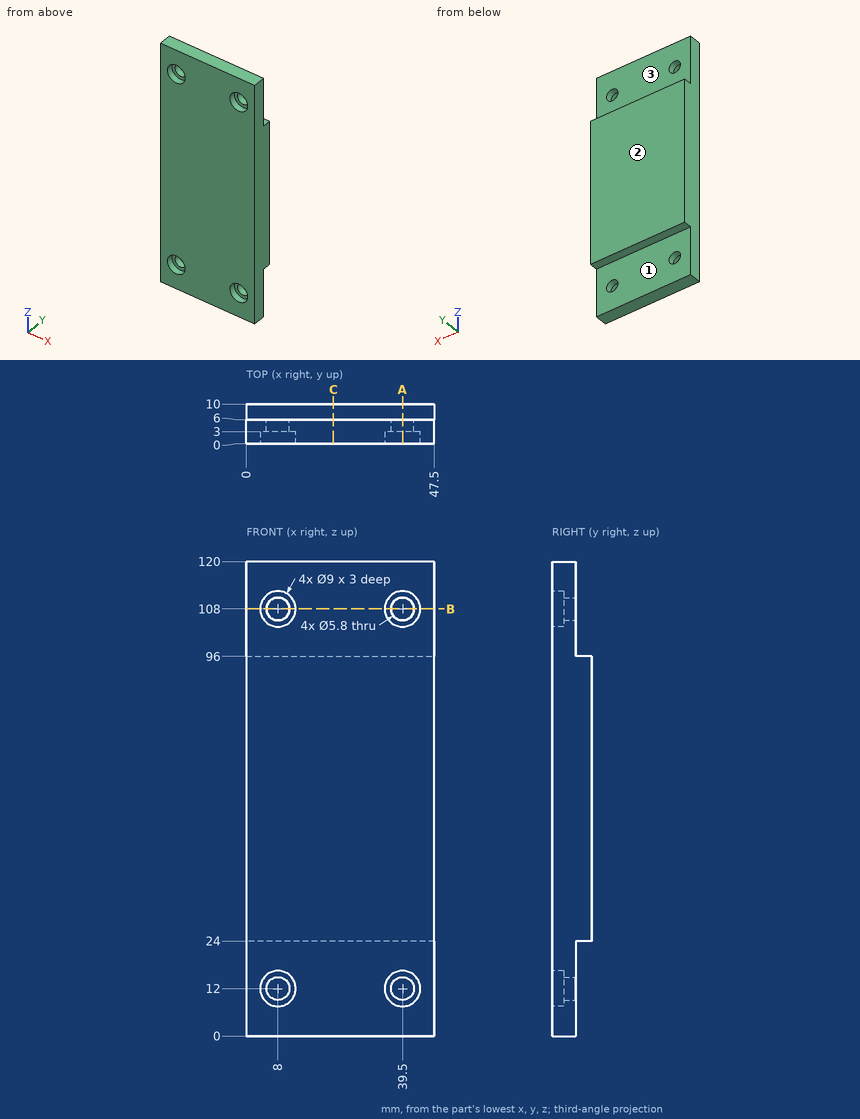
Job drawing, mm, ordinate dimensions from the low corner. One solid piece. A direction names the side the tool comes from. Coordinates: 2 decimals unless noted, no trailing zeros. Loops run counter-clockwise (first coordinate to the right, second up) from the corner with the lowest first, then second, coordinate; pieces in that order, holes last. Notation, with made-up numbers: (-1.5, 59.25) - (19.5, 59.25) arc R26 cw to (19.5, 90.25) - close; hole circle Ø2 at (65.5, 21.25). An arc over 180 degrees is marked (long way). Answer as a JSON object with one key per item and string values. Group by question number.
(1) Tool access for the marked faces 1, 2 and 3: list every direction of +Z, -Z, +X, -X, +Y, -Y with a clear straight run to the whole face (end or side of a thin tool).
(2) Cut at C-C (x = 22). Give the cut face in (y, z), then the cut area to 3 significant figures.
(3) Probe line 1 along X through (y, z) = (5.45, 108); line 2 along Z through (x, y) = (39.5, 1.95); line 3 along Z through (x, y) = (39.5, 4.95). List the from-to ranges inside material, lowest first.
(4) Cut at B-B (z = 108). Give the cut face in (x, y), then the cut area to 3 significant figures.
(5) Flat gauge pins, fed straight in: pin 1 (2.5 mm diameter, centred on x = 39.5, z = 106, fed in from -Y); pin 2 (2 mm diameter, centred on x = 17, y = 9, fed in from -Z); pin 3 (2.5 mm diameter, centred on x = 8, z = 13.5, fed in from -Y); pin 4 (12 mm diameter, centred on x = 22, z = 108, fed in from +Y). Where does each tip first touch, or does it go through?
(6) Cut at A-A (x = 39.5). Give the cut face in (y, z), then the cut area to 3 significant figures.
Geometry says:
{
 "1": {"face 1": "-Z, +X, -X, +Y", "face 2": "+Z, -Z, +X, -X, +Y", "face 3": "+Z, +X, -X, +Y"},
 "2": {"outline": "(0, 0) - (6, 0) - (6, 24) - (10, 24) - (10, 96) - (6, 96) - (6, 120) - (0, 120) - close", "area": "1,010 mm^2"},
 "3": {"line 1": "x = 0 to 5.1, 10.9 to 36.6, 42.4 to 47.5", "line 2": "z = 0 to 7.5, 16.5 to 103.5, 112.5 to 120", "line 3": "z = 0 to 9.1, 14.9 to 105.1, 110.9 to 120"},
 "4": {"outline": "(0, 0) - (3.5, 0) - (3.5, 3) - (5.1, 3) - (5.1, 6) - (0, 6) - close; (10.9, 3) - (12.5, 3) - (12.5, 0) - (35, 0) - (35, 3) - (36.6, 3) - (36.6, 6) - (10.9, 6) - close; (42.4, 3) - (44, 3) - (44, 0) - (47.5, 0) - (47.5, 6) - (42.4, 6) - close", "area": "196 mm^2"},
 "5": {"pin 1": "stops at y = 3", "pin 2": "stops at z = 24", "pin 3": "passes through", "pin 4": "stops at y = 6"},
 "6": {"outline": "(0, 0) - (6, 0) - (6, 9.1) - (3, 9.1) - (3, 7.5) - (0, 7.5) - close; (0, 16.5) - (3, 16.5) - (3, 14.9) - (6, 14.9) - (6, 24) - (10, 24) - (10, 96) - (6, 96) - (6, 105.1) - (3, 105.1) - (3, 103.5) - (0, 103.5) - close; (0, 112.5) - (3, 112.5) - (3, 110.9) - (6, 110.9) - (6, 120) - (0, 120) - close", "area": "919 mm^2"}
}
